Check sheet for the modelled part. Datum: model origin and axes. Units: mm. Round coordinates to 2 decimals unless told otherwise and drop trailing zeros. Order: outer loops, then holes, each group sorted by start corner. A loop starts at its lowest first (then second) coordinate and runs counter-clockwise, first axis right, second up.
Q1. Cross-section at A-A on y = 0.55. Record the cut outline in (x, z), then the cut area to 3 significant figures.
Q2. Cross-section at B-B on z = 6. Record the cut outline in (x, y), then the cut area to 3 significant figures.
Q3. Scan lines: probe 1 along Z at (x, y) = (-49.5, 0.75); probe 2 along X at (y, z) = (0.6, 13.5); probe 3 along X at (y, z) = (0.7, 21). Record each from-to range of solid material in increasing order.
Q4. Cross-section at C-C on x = -42.5. Record the cut outline in (y, z), then the cut area to 3 significant figures.
from build123d import *

# Parameters (mm, degrees)
EXTRUDE1_DEPTH = 1.6002


with BuildPart() as part:
    # Sketch1 → Extrude1 (new body)
    with BuildSketch(Plane(origin=(0, 0, 0), x_dir=(1, 0, 0), z_dir=(0, 1, 0))):
        with BuildLine():
            Line((21.182243879, 0), (-21.182243879, 0))
            ThreePointArc((-21.182243879, 0), (-23.612283674, -0.483364969), (-25.672371939, -1.859871939))
            Line((-25.672371939, -1.859871939), (-55.9435, -32.131))
            Line((-55.9435, -32.131), (55.9435, -32.131))
            Line((55.9435, -32.131), (25.672371939, -1.859871939))
            ThreePointArc((25.672371939, -1.859871939), (23.612283674, -0.483364969), (21.182243879, 0))
        make_face()
    extrude(amount=EXTRUDE1_DEPTH)


solid = part.part
Results found:
1. outline: (-55.94, 32.13) - (-25.67, 1.86) arc R6.35 ccw to (-21.18, 0) - (21.18, 0) arc R6.35 ccw to (25.67, 1.86) - (55.94, 32.13) - close
1. area: 2,560 mm2
2. outline: (-29.81, 0) - (29.81, 0) - (29.81, 1.6) - (-29.81, 1.6) - close
2. area: 95.4 mm2
3. probe 1: z = 25.69 to 32.13
3. probe 2: x = -37.31 to 37.31
3. probe 3: x = -44.81 to 44.81
4. outline: (0, 18.69) - (1.6, 18.69) - (1.6, 32.13) - (0, 32.13) - close
4. area: 21.5 mm2
